Geometry check sheet. Reference: drawing and pictorial views, mm from the part's lowest x, y, z. A direction names the side the tool comes from. Give positions to 0.01 mm unless a question says otherwise; leave off trailing zeros. Order: outer loops, then holes, each group sorted by start corner. A loop starts at its lowest first (then second) coordinate and runs counter-clockwise, first axis right, second up.
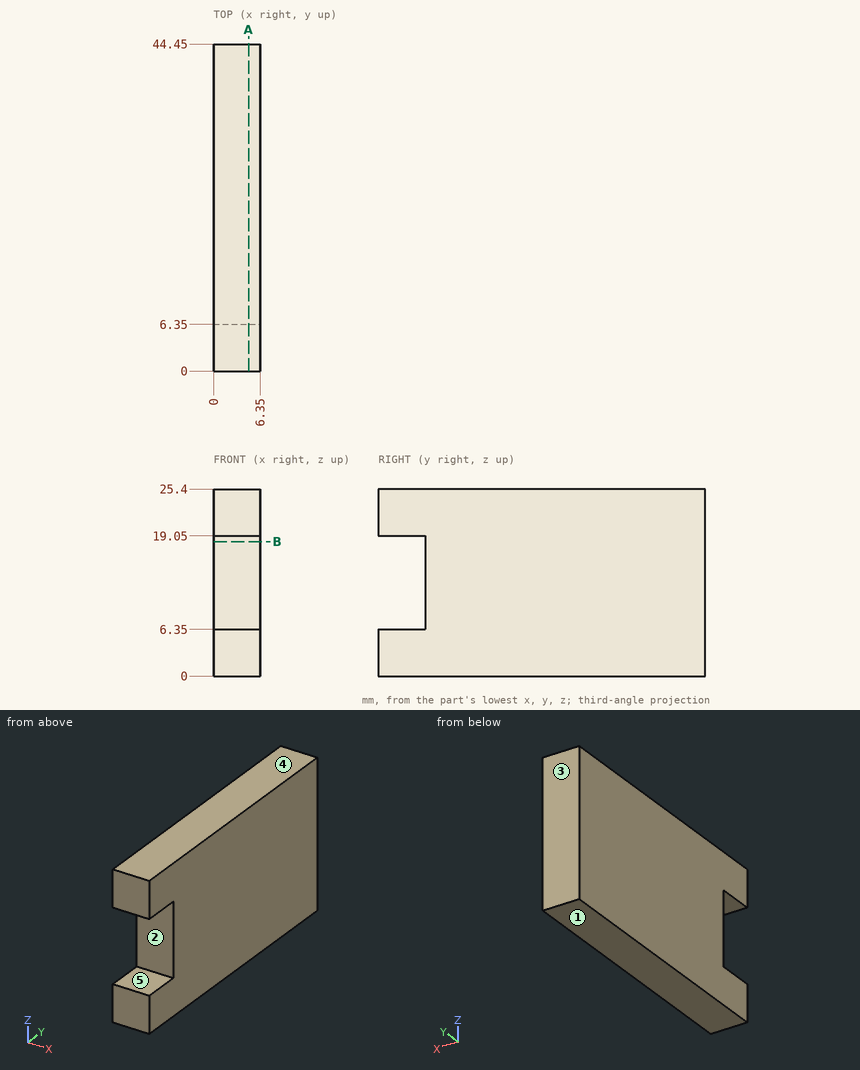
(1) Go/stop test with a flat-tipped pin: P1, Ø1.5, axis at x = 2, z = 12, coming from the -Y side. Record where the tip stops, or that it passes through.
(2) Thickness scan on L1, parallel to Y at x = 2.5, z = 8. Record the ranges inside material, lowest first.
(3) Sectioned sample at B-B (z = 18.25). Enter the section's corners in (x, y), plus the area to 3 significant figures.
(4) Tool access check on the marked faces 4 and 5. Record the directions out of +Z, -Z, +X, -X, +Y, -Y that give a thin tool (end or side, any length) a straight path to the whole face; none if there is none.
(5) Release check for a two-part mould opening along Z. For the marked faces 1, 2 and 3 record: released by +Z, released by -Z, zero draft, split by the parting line, or undercut.
(6) Sectioned sample at A-A (x = 4.75). Enter the section's corners in (y, z), plus the area to 3 significant figures.
Values follow:
1. P1: stops at y = 6.35
2. L1: y = 6.35 to 44.45
3. outline: (0, 6.35) - (6.35, 6.35) - (6.35, 44.45) - (0, 44.45) - close
3. area: 242 mm2
4. face 4: +Z, +X, -X, +Y, -Y
4. face 5: +X, -X, -Y
5. face 1: released by -Z
5. face 2: undercut
5. face 3: zero draft
6. outline: (0, 0) - (44.45, 0) - (44.45, 25.4) - (0, 25.4) - (0, 19.05) - (6.35, 19.05) - (6.35, 6.35) - (0, 6.35) - close
6. area: 1,050 mm2
